```python
from build123d import *

# Parameters (mm, degrees)
SKETCH1_W                  = 10
SKETCH1_H                  = 10
BOSS_EXTRUDE1_DEPTH        = 12
F_10_32_TAPPED_HOLE1_D     = 4.0386
F_10_32_TAPPED_HOLE1_DEPTH = 5
F_10_32_TAPPED_HOLE1_TIP   = 1.213317848
M2X0_4_TAPPED_HOLE1_D      = 1.6
M2X0_4_TAPPED_HOLE1_DEPTH  = 7
M2X0_4_TAPPED_HOLE1_TIP    = 0.480688495


with BuildPart() as part:
    # Sketch1 → Boss-Extrude1 (new body)
    with BuildSketch(Plane.XY):
        Rectangle(SKETCH1_W, SKETCH1_H)
    extrude(amount=BOSS_EXTRUDE1_DEPTH)

    # #10-32 Tapped Hole1
    with Locations(Plane(origin=(0, 0, 0), x_dir=(1, 0, 0), z_dir=(0, 0, -1))):
        with Locations((0, 0)):
            Hole(F_10_32_TAPPED_HOLE1_D / 2, depth=F_10_32_TAPPED_HOLE1_DEPTH)
            with Locations((0, 0, -(F_10_32_TAPPED_HOLE1_DEPTH + F_10_32_TAPPED_HOLE1_TIP / 2))):  # 118° drill point
                Cone(0, F_10_32_TAPPED_HOLE1_D / 2, F_10_32_TAPPED_HOLE1_TIP, mode=Mode.SUBTRACT)

    # M2x0.4 Tapped Hole1
    with Locations(Plane.XY.offset(12)):
        with Locations((0, 0)):
            Hole(M2X0_4_TAPPED_HOLE1_D / 2, depth=M2X0_4_TAPPED_HOLE1_DEPTH)
            with Locations((0, 0, -(M2X0_4_TAPPED_HOLE1_DEPTH + M2X0_4_TAPPED_HOLE1_TIP / 2))):  # 118° drill point
                Cone(0, M2X0_4_TAPPED_HOLE1_D / 2, M2X0_4_TAPPED_HOLE1_TIP, mode=Mode.SUBTRACT)


solid = part.part
```
Geometry: final body of the model. Coordinates: model frame, mm. Give positions to 0.01 mm unless a question says otherwise; leave off trailing zeros. Loops run counter-clockwise (first coordinate to the right, second up) from the corner with the lowest first, then second, coordinate; pieces in that order, holes last. Notation, with made-up numbers: (30, 11) -> (40, 11) arc R31 ccw to (40, 39) -> close; hole circle Ø10 at (18, 24). An arc over 180 degrees is marked (long way). Use one line per item in the form item = value.
Item 1: Section query C-C on z = 8.5. Output: boundary loops of the cut face in (x, y), and give its area (3 significant figures).
A:
outline = (-5, -5) -> (5, -5) -> (5, 5) -> (-5, 5) -> close; hole circle Ø1.6 at (0, 0)
area = 98.0 mm^2
Item 2: Section query D-D on z = 3.5. Output: boundary loops of the cut face in (x, y), and give its area (3 significant figures).
A:
outline = (-5, -5) -> (5, -5) -> (5, 5) -> (-5, 5) -> close; hole circle Ø4.04 at (0, 0)
area = 87.2 mm^2
Item 3: Section query A-A on x = 0. Output: boundary loops of the cut face in (y, z).
A:
outline = (-5, 0) -> (-2.02, 0) -> (-2.02, 5) -> (-0.8, 5.73) -> (-0.8, 12) -> (-5, 12) -> close; (0.8, 5.73) -> (2.02, 5) -> (2.02, 0) -> (5, 0) -> (5, 12) -> (0.8, 12) -> close
Item 4: Pin query (flat end, axial travel): P1, Ø2.5, axis at x = 0, y = 0, coming from the -Z side. Return the tip coordinate at first contact, or that it passes through.
A:
P1 = 5.46
Item 5: Draft query along X for faces 1 (the face through (2.2, 0.1, 0)), 2 (the face through (5, 0, 6)), 3 (the face through (-1.926, -0.607, 2.535)), 4 (the face through (-5, 0, 6)). Return one class per face: pulls with the +X half, pulls with the -X half, needs draft (parallel to the pull), parting line crosses it, or undercut.
A:
face_1 = needs draft
face_2 = pulls with the +X half
face_3 = undercut
face_4 = pulls with the -X half
Item 6: Line query: probe 1 along Y at (x, z) = (0, 2.05); probe 2 along Y at (x, z) = (0, 8); probe 3 along X at (y, z) = (-1.75, 4.75). Output: solid intervals per line, ascending.
A:
probe_1 = -5 to -2.02, 2.02 to 5
probe_2 = -5 to -0.8, 0.8 to 5
probe_3 = -5 to -1.01, 1.01 to 5
